from build123d import *

# Parameters (mm, degrees)
REVOLVE1_ANGLE     = 180
SKETCH2_R          = 10.45
CUT_EXTRUDE1_DEPTH = 169.759266412
SKETCH3_R          = 1
CUT_EXTRUDE2_DEPTH = 169.759266558
CIRPATTERN1_COUNT  = 4


with BuildPart() as part:
    # Sketch1 → Revolve1 (revolve)
    with BuildSketch(Plane.XY):
        Polygon((-45, 0), (-45, 156.3), (-43, 156.3), (-43, 141.3), (-41, 141.3), (-41, 15), (-43, 15), (-43, 0), align=None)
    revolve(axis=Axis((0, 0, 0), (0, 1, 0)), revolution_arc=REVOLVE1_ANGLE)

    # Sketch2 → Cut-Extrude1 (cut, through all)
    with BuildSketch(Plane(origin=(0, 0, 0), x_dir=(0, 0, -1), z_dir=(1, 0, 0))):
        with Locations((0, 40.3)):
            Circle(SKETCH2_R)
        with Locations((0, 91.5)):
            Circle(SKETCH2_R)
    extrude(amount=-CUT_EXTRUDE1_DEPTH, mode=Mode.SUBTRACT)

    # Sketch3 → Cut-Extrude2 (cut, through all)
    with BuildSketch(Plane(origin=(0, 0, 0), x_dir=(0, 1, 0), z_dir=(0.7071067811865464, 0, -0.7071067811865488))):
        with Locations(Location((7.5, 0, 0), (0, 0, 270))):
            Circle(SKETCH3_R)
        with Locations(Location((148.8, 0, 0), (0, 0, 270))):
            Circle(SKETCH3_R)
    cut_extrude2 = extrude(amount=-CUT_EXTRUDE2_DEPTH, mode=Mode.SUBTRACT)

    # CirPattern1: Cut-Extrude2 ×4 about axis
    cirpattern1_axis = Axis((0, 0, 0), (0, -1, 0))
    for i in range(1, CIRPATTERN1_COUNT):
        add(cut_extrude2.rotate(cirpattern1_axis, i * 360 / CIRPATTERN1_COUNT), mode=Mode.SUBTRACT)


solid = part.part
Source: CAD feature listing. Evaluate the final solid. Frame: model axes, mm. A direction names the side the tool comes from. Coordinates: 2 decimals unless noted, no trailing zeros. Loops run counter-clockwise (first coordinate to the right, second up) from the corner with the lowest first, then second, coordinate; pieces in that order, holes last. Notation, with made-up numbers: (61, -32) - (104, -32) arc R17 ccw to (104, -2) - close; hole circle Ø10 at (-31, 62). An arc over 180 degrees is marked (long way). One line per item, written item: value. Start each with the question number.
1. Section C-C (x = 0). Return the cut outline in (y, z), and give its area (3 significant figures).
2. Section A-A (z = 15). Return the cut outline in (x, y).
3. Set-up query: faces 1 (the flat face through (-6, 141.3, 41)), 2 (the cylindrical face through (-42.285, 40.53, 10.447)), 3 (the cylindrical face through (-0.95, 7.4, 42.99)). Return all of +Z, -Z, +X, -X, +Y, -Y with unobstructed straight access to the full face (end or side cutting, diameter ignored); none if empty.
4. Section D-D (y = 23). Return the cut outline in (x, z), and give its area (3 significant figures).
5. Contact query for flat-ended pins moving along their axis: P1, Ø10, axis at x = -10.5, y = 34.5, coming from the +Z side; P2, Ø1.5, axis at x = 13, y = 83, coming from the -Z side; P3, Ø5, axis at x = 1, z = 40, coming from the -Y side. Output: stop coordinate, or through.
6. Ray query, L1, parallel to X at y = 119.5, z = 30; L2, parallel to X at y = 65, z = 17; L3, parallel to Z at x = -1.5, y = 107 (3 decimals). Return the intervals inside material, ascending.
7. Section B-B (z = 8). Return the cut outline in (x, y).
8. Mould query, pull axis Y, two halves, no side actions, for faces 4 (the flat face through (-43, 18, 0)), 5 (the flat face through (-6, 156.3, 43)), 6 (the cylindrical face through (31.19, 149.79, 31.01)), 7 (the flat face through (6, 0, 43)). Classes: pulls with the +Y half, pulls with the -Y half, needs draft (parallel to the pull), parting line crosses it, or undercut.
Verdict:
1. outline: (0, 43) - (15, 43) - (15, 41) - (141.3, 41) - (141.3, 43) - (156.3, 43) - (156.3, 45) - (0, 45) - close
1. area: 565 mm2
2. outline: (-42.43, 0) - (-40.3, 0) - (-40.3, 15) - (-38.16, 15) - (-38.16, 141.3) - (-40.3, 141.3) - (-40.3, 156.3) - (-42.43, 156.3) - close; (38.16, 15) - (40.3, 15) - (40.3, 0) - (42.43, 0) - (42.43, 156.3) - (40.3, 156.3) - (40.3, 141.3) - (38.16, 141.3) - close
3. face 1: -Z, +Y
3. face 2: -Z, -X
3. face 3: -Z, -Y
4. outline: (-45, 0) - (-41, 0) arc R41 cw to (41, 0) - (45, 0) arc R45 ccw to start
4. area: 540 mm2
5. P1: stops at z = 44.66
5. P2: stops at z = 38.63
5. P3: stops at y = 15
6. L1: x = -33.54 to -27.95, 27.95 to 33.54
6. L2: x = -41.67 to -37.31, 37.31 to 41.67
6. L3: z = 40.973 to 44.975
7. outline: (-44.28, 0) - (-42.25, 0) - (-42.25, 15) - (-40.21, 15) - (-40.21, 33.58) - (-44.28, 33.58) - close; (-44.28, 47.02) - (-40.21, 47.02) - (-40.21, 84.78) - (-44.28, 84.78) - close; (-44.28, 98.22) - (-40.21, 98.22) - (-40.21, 141.3) - (-42.25, 141.3) - (-42.25, 156.3) - (-44.28, 156.3) - close; (40.21, 15) - (42.25, 15) - (42.25, 0) - (44.28, 0) - (44.28, 156.3) - (42.25, 156.3) - (42.25, 141.3) - (40.21, 141.3) - close
8. face 4: needs draft
8. face 5: pulls with the +Y half
8. face 6: undercut
8. face 7: pulls with the -Y half
